```python
from build123d import *

# Parameters (mm, degrees)
BOSS_EXTRUDE1_DEPTH              = 12.7
F_1_4_CLEARANCE_HOLE1_D          = 6.7564
F_1_4_CLEARANCE_HOLE1_DEPTH      = 6.35
SKETCH4_W                        = 3.3782
SKETCH4_H                        = 6.35
F_1_4_CLEARANCE_HOLE2_AT_2_COUNT = 2
F_1_4_CLEARANCE_HOLE2_AT_2_PITCH = 25.4
SKETCH6_R                        = 4.7625
CUT_EXTRUDE1_DEPTH               = 70.85
SKETCH7_R                        = 4.7625
CUT_EXTRUDE2_DEPTH               = 58.15


with BuildPart() as part:
    # Sketch1 → Boss-Extrude1 (new body)
    with BuildSketch(Plane.XY):
        Polygon((0, 0), (0, 63.5), (76.2, 0), align=None)
        Polygon((6.35, 49.94248576), (6.35, 6.35), (58.660982912, 6.35), align=None, mode=Mode.SUBTRACT)
    extrude(amount=BOSS_EXTRUDE1_DEPTH)

    # 1/4 Clearance Hole1
    with Locations(Plane(origin=(6.35, 0, 0), x_dir=(0, 0, -1), z_dir=(1, 0, 0))):
        with Locations((-6.35, 12.7), (-6.35, 38.1)):
            Hole(F_1_4_CLEARANCE_HOLE1_D / 2, depth=F_1_4_CLEARANCE_HOLE1_DEPTH)

    # Sketch4 → 1/4 Clearance Hole2 (revolve, cut)
    with BuildSketch(Plane(origin=(25.4, 6.35, 6.35), x_dir=(0, 0, 1), z_dir=(1, 0, 0))):
        with Locations((1.6891, 3.175)):
            Rectangle(SKETCH4_W, SKETCH4_H)
    f_1_4_clearance_hole2 = revolve(axis=Axis((25.4, 12.7, 6.35), (0, -1, 0)), mode=Mode.SUBTRACT)

    # 1/4 Clearance Hole2 at 2: 1/4 Clearance Hole2 ×2
    with Locations(*[(i * F_1_4_CLEARANCE_HOLE2_AT_2_PITCH, 0, 0) for i in range(1, F_1_4_CLEARANCE_HOLE2_AT_2_COUNT)]):
        add(f_1_4_clearance_hole2, mode=Mode.SUBTRACT)

    # Sketch6 → Cut-Extrude1 (cut, through all)
    with BuildSketch(Plane(origin=(6.35, 0, 0), x_dir=(0, 0, -1), z_dir=(1, 0, 0))):
        with Locations((-6.35, 38.1)):
            Circle(SKETCH6_R)
    extrude(amount=CUT_EXTRUDE1_DEPTH, mode=Mode.SUBTRACT)

    # Sketch7 → Cut-Extrude2 (cut, through all)
    with BuildSketch(Plane(origin=(0, 6.35, 0), x_dir=(1, 0, 0), z_dir=(0, 1, 0))):
        with Locations((50.8, -6.35)):
            Circle(SKETCH7_R)
    extrude(amount=CUT_EXTRUDE2_DEPTH, mode=Mode.SUBTRACT)


solid = part.part
```
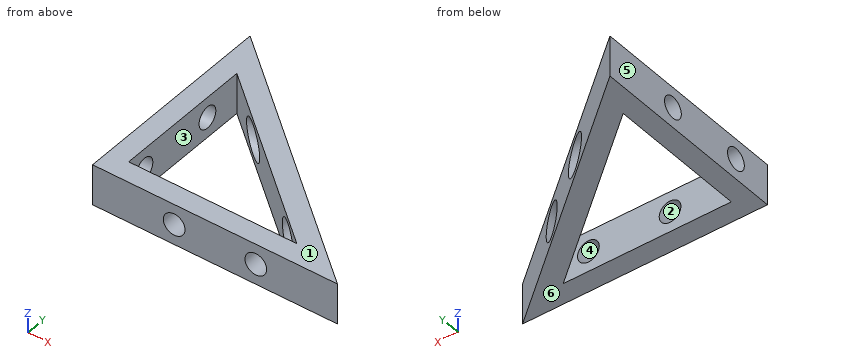
Input: part model. Units: mm. Frame: model coordinates. Face numbers are marked on the shaded views. A direction names the side the tool comes from. Coordinates: 2 decimals unless noted, no trailing zeros. Order: outer loops, then holes, each group sorted by start corner. A loop starts at its lowest first (then second) coordinate and runs counter-clockwise, first axis right, second up. Notation, with made-up numbers: (1, -28.5) - (33, -28.5) arc R17 ccw to (33, -20.5) - close; hole circle Ø6 at (68.25, 88). An arc over 180 degrees is marked (long way). Return JSON: item names as keys, results as strings.
Q1. Cut plane C-C (y = 39.5). Return loops of the section in (x, z), then the cut area to 3 significant figures.
The answers:
{"outline": "(0, 0) - (6.35, 0) - (6.35, 3.28) - (0, 3.28) - close; (0, 9.42) - (6.35, 9.42) - (6.35, 12.7) - (0, 12.7) - close; (18.88, 0) - (28.8, 0) - (28.8, 1.8) - (18.88, 1.8) - close; (18.88, 10.9) - (28.8, 10.9) - (28.8, 12.7) - (18.88, 12.7) - close", "area": "77.3 mm2"}
Q2. First-contact query: pin 1 (6 mm diameter, centred on x = 50.8, z = 6.35, fed in from -Y); pin 2 (4 mm diameter, centred on y = 24.5, z = 9.5, fed in from +X); pin 3 (1 mm diameter, centred on x = 67, z = 6.5, fed in from +Y); pin 4 (6.5 mm diameter, centred on x = 39.5, z = 3.5, fed in from +Y). Flat tips, straight axial feed; report the tip coordinate or a pass-through.
The answers:
{"pin 1": "passes through", "pin 2": "stops at x = 48.76", "pin 3": "stops at y = 8.08", "pin 4": "stops at y = 33.29"}
Q3. Ray query, probe 1 along Z at (x, y) = (29.75, 38.1); probe 2 along Y at (x, z) = (3, 6.35); probe 3 along Y at (x, z) = (3.5, 4.25). Return the intervals inside material, ascending.
The answers:
{"probe 1": "z = 0 to 1.59, 11.11 to 12.7", "probe 2": "y = 0 to 9.32, 16.08 to 34.72, 41.48 to 61", "probe 3": "y = 0 to 10.05, 15.35 to 35.45, 40.75 to 60.58"}
Q4. Draft query along Z for the marked faces 4, 5 and 6. Return one class per face: +Z half, -Z half, draft (parallel to the pull), parting line (faces both ways), or undercut.
The answers:
{"face 4": "undercut", "face 5": "draft", "face 6": "-Z half"}
Q5. Access query for the marked faces 1, 2 and 3. Directions: +Z, -Z, +X, -X, +Y, -Y. A direction counts if a zero-diameter tool reaches every point of the face in a straight line with its end or side. Return the directions, or none.
The answers:
{"face 1": "+Z, +X, -X, +Y, -Y", "face 2": "-Y", "face 3": "+Z, -Z"}
Q6. Cut plane A-A (z = 4.25). State how many separate pieces and enclosed holes the cut face has, then the cut area to 3 significant figures.
The answers:
{"separate pieces": "6", "enclosed holes": "0", "area": "989 mm2"}
Q7. Cut plane D-D (x = 42). Return loops of the section in (y, z).
The answers:
{"outline": "(0, 0) - (6.35, 0) - (6.35, 12.7) - (0, 12.7) - close; (20.23, 0) - (28.5, 0) - (28.5, 12.7) - (20.23, 12.7) - close"}
